Autodesk Inventor part; units mm, degrees
ref_plane "YZ Plane" through (0, 0, 0) normal (1, 0, 0) x (0, 1, 0)
ref_plane "XZ Plane" through (0, 0, 0) normal (0, 1, 0) x (-1, 0, 0)
ref_plane "XY Plane" through (0, 0, 0) normal (0, 0, 1) x (1, 0, 0)
sketch "Boceto1" plane through (0, 0, 0) normal (0, 1, 0) x (-1, 0, 0)
  line L0 (53, 63) -> (-53, 63)
  line L1 (-53, 63) -> (-53, -63)
  line L2 (-53, -63) -> (53, -63)
  line L3 (53, -63) -> (53, 63)
  point P0 (0, 0)
  point P1 (0, 63)
  dimension "d1" = 106
  dimension "d2" = 126
  dimension "d3" = 53
  dimension "d4" = 63
extrude "Extrusión1" add sketch "Boceto1" along normal blind 5
sketch "Boceto2" plane through (0, 5, 0) normal (0, 1, 0) x (1, 0, 0)
  circle A0 centre (-45.929, -42.384) radius 1.5
  line L0 (-53, -63) -> (53, -63)
  line L1 (-53, 63) -> (-53, -63)
  line L2 (-81, 0) -> (77, 0)
  line L3 (0, -130) -> (0, 128)
  circle A1 centre (-45.929, 42.384) radius 1.5
  line L4 (-53, -63) -> (-53, 63)
  circle A2 centre (45.929, -42.384) radius 1.5
  circle A3 centre (45.929, 42.384) radius 1.5
  point P0 (0, 0)
  dimension "d7" = 3
  dimension "d8" = 20.616
  dimension "d9" = 7.071
extrude "Extrusión2" add sketch "Boceto2" along normal blind 10 contours A0 | A1 | A2 | A3
sketch "Boceto3" plane through (0, 0, 0) normal (0, -1, 0) x (1, 0, 0)
  line L0 (-35, 52.5) -> (35, 52.5)
  line L1 (35, 52.5) -> (35, -52.5)
  line L2 (35, -52.5) -> (-35, -52.5)
  line L3 (-35, -52.5) -> (-35, 52.5)
  line L4 (53, -63) -> (-53, -63)
  line L5 (-53, 63) -> (53, 63)
  line L6 (53, 63) -> (53, -63)
  line L7 (-53, -63) -> (-53, 63)
  line L8 (35, 17.5) -> (-35, 17.5)
  line L9 (35, -17.5) -> (-35, -17.5)
  line L10 (0, 52.5) -> (0, -52.5)
  point P0 (0, 0)
  point P1 (0, 17.5)
  dimension "d12" = 52.5
  dimension "d13" = 126
  dimension "d14" = 106
  dimension "d15" = 52.5
  dimension "d16" = 35
  dimension "d17" = 35
  dimension "d18" = 35
  dimension "d19" = 35
  dimension "d20" = 35
extrude "Extrusión3" cut sketch "Boceto3" against normal blind 2 contours L0 L10 L8 L3 | L0 L1 L8 L10
properties part number "Tapa 0"
The listing builds one solid part. Answer for the finished solid, in the listing's coordinates (mm). A direction names the side the tool comes from. Round coordinates to 2 decimals unless told otherwise and drop trailing zeros. Write each loop counter-clockwise with the first axis right and the second up, starting at its lowest first coordinate (ties: lowest second). Pieces come first, ordered by that corner, then holes. Notation, with made-up numbers: (77.5, 78) - (122.5, 78) arc R16 ccw to (122.5, 108) - close; hole circle Ø4 at (37.5, 71). An arc over 180 degrees is marked (long way). Use a Markdown table: item, result. Add a question column.
1. The part is cut by section A-A (x = -32). Write down the section's boundary in (y, z), and give its area (3 significant figures).
2. Consider line 1 (Y direction, x = 3, z = -31.5); line 2 (Y direction, x = 16, z = 38); line 3 (Z direction, x = 45.5, y = 13.75). Determine where each line is inside the solid, lowest interval first.
3. A tool of negligible diameter and unlimited length cuts with its end or side. For faces 1 (the face through (53, 2, 1)), 2 (the face through (0, 2, 35)), 3 (the face through (46.621, 9.93, -43.715)), from which of +Z, -Z, +X, -X, +Y, -Y can it reach the whole face along a straight path? Write none if from no direction.
4. For a pull along X with two mould halves and no side action, classify faces 4 (the face through (46.621, 9.93, 41.053)), 5 (the face through (-53, 2, -1)), 6 (the face through (46, 15, -42)), 7 (the face through (-47.12, 9.93, 41.47)) as +X half, -X half, draft (parallel to the pull), parting line (faces both ways), or undercut.
5. The part is cut by section D-D (z = -13). Write down the section's boundary in (x, y), and give its area (3 significant figures).
6. The part is cut by section B-B (z = 23). Write down the section's boundary in (x, y).
7. The part is cut by section C-C (y = 10.5). Write down the section's boundary in (x, z).
Reported:
| question | item | result |
|---|---|---|
| 1 | outline | (0, -63) - (5, -63) - (5, 63) - (0, 63) - (0, 52.5) - (2, 52.5) - (2, 17.5) - (0, 17.5) - close |
| 1 | area | 560 mm^2 |
| 2 | line 1 | 0 to 5 |
| 2 | line 2 | 2 to 5 |
| 2 | line 3 | -43.82 to -40.95, 40.95 to 43.82 |
| 3 | face 1 | +Z, -Z, +X, +Y, -Y |
| 3 | face 2 | -Y |
| 3 | face 3 | +Y |
| 4 | face 4 | undercut |
| 4 | face 5 | -X half |
| 4 | face 6 | draft |
| 4 | face 7 | undercut |
| 5 | outline | (-53, 0) - (53, 0) - (53, 5) - (-53, 5) - close |
| 5 | area | 530 mm^2 |
| 6 | outline | (-53, 0) - (-35, 0) - (-35, 2) - (35, 2) - (35, 0) - (53, 0) - (53, 5) - (-53, 5) - close |
| 7 | outline | circle Ø3 at (-45.93, -42.38); circle Ø3 at (-45.93, 42.38); circle Ø3 at (45.93, -42.38); circle Ø3 at (45.93, 42.38) |
